Read the model definition and answer for the solid it produces. Units are mm, in the model's axes. A direction names the side the tool comes from. Give positions to 0.01 mm unless a question says otherwise; leave off trailing zeros. Write each loop counter-clockwise with the first axis right and the second up, starting at its lowest first coordinate (ties: lowest second). Pieces come first, ordered by that corner, then holes. Notation, with made-up numbers: M -34.5,2 L 9.5,2 A23 cw 9.5,13 Z; hole C -31.5,51.25 d9. An arc over 180 degrees is marked long. Put each result on its own line as item: value.
Autodesk Fusion 360 part; units mm, degrees
sketch "Sketch2" plane through (0, 0, 0) normal (0, 0, 1) x (1, 0, 0)
  line L0 (0, 0) -> (79, 0)
  line L1 (79, 0) -> (79, 44)
  line L2 (79, 44) -> (0, 44)
  line L3 (0, 44) -> (0, 0)
  line L4 (1.2, 1.2) -> (77.8, 1.2)
  line L5 (77.8, 1.2) -> (77.8, 42.8)
  line L6 (77.8, 42.8) -> (1.2, 42.8)
  line L7 (1.2, 42.8) -> (1.2, 1.2)
  circle A0 centre (5, 39) radius 1.6
  line L8 (6.5877, 41.75) -> (3.4123, 41.75)
  line L9 (3.4123, 41.75) -> (1.8246, 39)
  line L10 (1.8246, 39) -> (3.4123, 36.25)
  line L11 (3.4123, 36.25) -> (6.5877, 36.25)
  line L12 (6.5877, 36.25) -> (8.1754, 39)
  line L13 (8.1754, 39) -> (6.5877, 41.75)
  line L14 (2, 2) -> (77, 2)
  line L15 (77, 2) -> (77, 42)
  line L16 (77, 42) -> (2, 42)
  line L17 (2, 42) -> (2, 2)
  line L18 (3.4, 41.75) -> (3.4, 36.25)
  line L19 (6.6, 41.75) -> (6.6, 36.25)
  line L20 (3.4, 40.6) -> (6.6, 40.6)
  line L21 (3.4, 37.4) -> (6.6, 37.4)
  circle A1 centre (74, 5) radius 1.6
  line L22 (75.5877, 7.75) -> (72.4123, 7.75)
  line L23 (72.4123, 7.75) -> (70.8246, 5)
  line L24 (70.8246, 5) -> (72.4123, 2.25)
  line L25 (72.4123, 2.25) -> (75.5877, 2.25)
  line L26 (75.5877, 2.25) -> (77.1754, 5)
  line L27 (77.1754, 5) -> (75.5877, 7.75)
  line L28 (72.4, 7.75) -> (72.4, 2.25)
  line L29 (75.6, 7.75) -> (75.6, 2.25)
  line L30 (71.7483, 6.6) -> (76.2517, 6.6)
  line L31 (71.7483, 3.4) -> (76.2517, 3.4)
  point P0 (5, 39)
  point P1 (74, 5)
  dimension "d48" = 44
  dimension "d49" = 79
  dimension "d50" = -1.2
  dimension "d55" = 3.2
  dimension "d56" = 3.8
  dimension "d57" = 3.8
  dimension "d58" = 2.75
  dimension "d59" = -2
  dimension "d60" = 3.2
  dimension "d61" = 3
  dimension "d62" = 3
  dimension "d63" = 2.75
extrude "Extrude10" add sketch "Sketch2" along normal blind 13.5 contours L0 L1 L2 L3
extrude "Extrude11" add sketch "Sketch2" along normal blind 9.8 contours L4 L5 L6 L7 | A0 | A0 L19 L21 | A0 L19 L20 | L12 L13 L19 | A0 L18 L20 | L8 L9 L13 L18 L19 L20 | A0 L18 L21 | L10 L11 L12 L18 L19 L21 | L9 L10 L17 L18 | L8 L9 L10 L11 L12 L13 L14 L15 L16 L17 L22 L23 L24 L25 L26 L27 | L9 L10 L17 | L15 L26 L27 | L15 L26 L27 L29 L30 L31 | L27 L29 L30 | L26 L29 L31 | L22 L23 L27 L28 L29 L30 | A1 L29 L30 | L24 L25 L26 L28 L29 L31 | A1 L29 L31 | A1 | A1 L28 L30 | A1 L28 L31 | L23 L24 L28 L30 L31 | L23 L28 L30 | L24 L28 L31
ref_plane "WorkPlane2" through (39.5, 22, 9.5) normal (0, 0, 1) x (1, 0, 0)
sketch "Sketch4" plane through (0, 0, 9.5) normal (0, 0, 1) x (1, 0, 0)
  line L0 (3.4, 41.75) -> (3.4, 36.25)
  line L1 (6.5877, 41.75) -> (3.4123, 41.75)
  line L2 (3.4, 40.6) -> (6.6, 40.6)
  line L3 (3.4123, 41.75) -> (1.8246, 39)
  line L4 (1.8246, 39) -> (3.4123, 36.25)
  circle A0 centre (5, 39) radius 1.6
  line L5 (3.4, 37.4) -> (6.6, 37.4)
  line L6 (3.4123, 36.25) -> (6.5877, 36.25)
  line L7 (6.6, 41.75) -> (6.6, 36.25)
  line L8 (8.1754, 39) -> (6.5877, 41.75)
  line L9 (6.5877, 36.25) -> (8.1754, 39)
  line L10 (75.5877, 7.75) -> (72.4123, 7.75)
  line L11 (72.4, 7.75) -> (72.4, 2.25)
  line L12 (71.7483, 6.6) -> (76.2517, 6.6)
  line L13 (72.4123, 7.75) -> (70.8246, 5)
  line L14 (70.8246, 5) -> (72.4123, 2.25)
  line L15 (71.7483, 3.4) -> (76.2517, 3.4)
  circle A1 centre (74, 5) radius 1.6
  line L16 (72.4123, 2.25) -> (75.5877, 2.25)
  line L17 (75.6, 7.75) -> (75.6, 2.25)
  line L18 (77.1754, 5) -> (75.5877, 7.75)
  line L19 (75.5877, 2.25) -> (77.1754, 5)
  line L20 (2, 42) -> (2, 2)
  line L21 (77, 42) -> (2, 42)
  line L22 (2, 2) -> (77, 2)
  line L23 (77, 2) -> (77, 42)
  line L24 (77.8, 42.8) -> (1.2, 42.8)
  line L25 (77.8, 1.2) -> (77.8, 42.8)
  line L26 (1.2, 1.2) -> (77.8, 1.2)
  line L27 (1.2, 42.8) -> (1.2, 1.2)
  line L28 (0, 0) -> (79, 0)
  line L29 (0, 44) -> (0, 0)
  line L30 (79, 0) -> (79, 44)
  line L31 (79, 44) -> (0, 44)
  line L32 (1.2, 42.8) -> (8.8, 42.8)
  line L33 (8.8, 42.8) -> (8.8, 35.2)
  line L34 (8.8, 35.2) -> (1.2, 35.2)
  line L35 (1.2, 35.2) -> (1.2, 42.8)
  line L36 (77.8, 1.2) -> (70.2, 1.2)
  line L37 (70.2, 1.2) -> (70.2, 8.8)
  line L38 (70.2, 8.8) -> (77.8, 8.8)
  line L39 (77.8, 8.8) -> (77.8, 1.2)
  dimension "d90" = 7.6
  dimension "d91" = 7.6
  dimension "d92" = 7.6
  dimension "d93" = 7.6
extrude "Extrude12" cut sketch "Sketch2" along normal blind 14 contours A0
extrude "Extrude13" cut sketch "Sketch2" along normal blind 8.7 contours A0 L19 L21 | A0 L19 L20 | A0 L18 L20 | A0 L18 L21
extrude "Extrude14" cut sketch "Sketch2" along normal blind 8.4 contours L8 L9 L13 L18 L19 L20 | L10 L11 L12 L18 L19 L21
extrude "Extrude15" cut sketch "Sketch2" along normal blind 8.1 contours L12 L13 L19 | L9 L10 L17 L18
extrude "Extrude16" cut sketch "Sketch2" along normal blind 8.1 contours L9 L10 L17
extrude "Extrude17" cut sketch "Sketch2" along normal blind 8.1 contours L15 L26 L27 | L15 L26 L27 L29 L30 L31 | L27 L29 L30 | L26 L29 L31 | L23 L24 L28 L30 L31 | L23 L28 L30 | L24 L28 L31
extrude "Extrude18" cut sketch "Sketch2" along normal blind 8.4 contours L22 L23 L27 L28 L29 L30 | L24 L25 L26 L28 L29 L31
extrude "Extrude19" cut sketch "Sketch2" along normal blind 8.7 contours A1 L29 L30 | A1 L29 L31 | A1 L28 L30 | A1 L28 L31
extrude "Extrude20" cut sketch "Sketch2" along normal blind 14 contours A1
ref_plane "WorkPlane3" through (39.5, 22, 9.8) normal (0, 0, 1) x (1, 0, 0)
sketch "Sketch5" plane through (0, 0, 9.8) normal (0, 0, 1) x (1, 0, 0)
  line L0 (70.2, 8.8) -> (77.8, 8.8)
  line L1 (70.2, 1.2) -> (70.2, 8.8)
  line L2 (77.8, 1.2) -> (70.2, 1.2)
  line L3 (77.8, 8.8) -> (77.8, 1.2)
  line L4 (8.8, 35.2) -> (1.2, 35.2)
  line L5 (8.8, 42.8) -> (8.8, 35.2)
  line L6 (1.2, 35.2) -> (1.2, 42.8)
  line L7 (1.2, 42.8) -> (8.8, 42.8)
  circle A0 centre (5, 39) radius 1.6
  circle A1 centre (74, 5) radius 1.6
extrude "Extrude22" add sketch "Sketch5" along normal blind 2.1 contours L4 L5 L6 L7
extrude "Extrude23" add sketch "Sketch5" along normal blind 2.1 contours L0 L1 L2 L3
(1) Section C-C on y = 10 is taken. Determine the outline of the cut face in (x, z), and give its area (3 significant figures).
Result:
outline: M 0,0 L 79,0 L 79,13.5 L 77.8,13.5 L 77.8,9.8 L 1.2,9.8 L 1.2,13.5 L 0,13.5 Z
area: 783 mm²
(2) Which of the six approach directions +Z, -Z, +X, -X, +Y, -Y give full straight-line access (tool end or side, diameter ignored) to faces 5 (the face through (7, 39, 8.1)), 6 (the face through (0, 22, 7)), 7 (the face through (1.2, 22, 12))?
Result:
face 5: -Z
face 6: +Z, -Z, -X, +Y, -Y
face 7: +Z
(3) For a pull along X with two mould halves and no side action, classify faces 1 (the face through (7.39, 40.36, 4.14)), 2 (the face through (3.7, 40.2, 8.7)), 3 (the face through (79, 22, 7)), 4 (the face through (39, 0, 7)) as +X half, -X half, draft (parallel to the pull), parting line (faces both ways), or undercut.
Result:
face 1: undercut
face 2: undercut
face 3: +X half
face 4: draft
(4) Straight lines are drawn through the part: line 1 along X through (y, z) = (39, 9.95); line 2 along X through (y, z) = (5, 11.05); line 3 along Y through (x, z) = (5, 9.9). For each, find the intervals that lie inside material, in ascending order. Write a range as from..to.
Result:
line 1: x = 0..3.4, 6.6..8.8, 77.8..79
line 2: x = 0..1.2, 70.2..72.4, 75.6..79
line 3: y = 0..1.2, 35.2..37.4, 40.6..44
(5) Section B-B on z = 7 is taken. Determine the outline of the cut face in (x, y), and give its area (3 significant figures).
Result:
outline: M 0,0 L 79,0 L 79,44 L 0,44 Z; hole M 1.82,39 L 3.41,36.25 L 6.59,36.25 L 8.18,39 L 6.59,41.75 L 3.41,41.75 Z; hole M 70.82,5 L 72.41,2.25 L 75.59,2.25 L 77.18,5 L 75.59,7.75 L 72.41,7.75 Z
area: 3,420 mm²
(6) Section A-A on x = 57 is taken. Determine the outline of the cut face in (y, z), and give its area (3 significant figures).
Result:
outline: M 0,0 L 44,0 L 44,13.5 L 42.8,13.5 L 42.8,9.8 L 1.2,9.8 L 1.2,13.5 L 0,13.5 Z
area: 440 mm²
(7) Given pin 1 Ø1.3 at (x, y) = (4, 38.5) entering from -Z; pin 2 Ø1.5 at (x, z) = (53, 9) entering from -Y; pin 3 Ø2 at (x, y) = (37, 39) entering from +Z, each flat-ended and moving along its own axis, determine where each tip first touches the part or whether it passes through.
Result:
pin 1: stops at z = 8.1
pin 2: stops at y = 0
pin 3: stops at z = 9.8
